Source: CAD feature listing. Evaluate the final solid. Frame: model axes, mm. Face numbers are marked on the shaded views. A direction names the side the tool comes from. Give positions to 0.01 mm unless a question says otherwise; leave off trailing zeros. Write each loop counter-clockwise with the first axis right and the second up, starting at its lowest first coordinate (ties: lowest second). Pieces come first, ordered by that corner, then holes. Notation, with made-up numbers: M 40.25,69 L 69.25,69 A31 ccw 69.25,105 Z; hole C 72.5,4 d4. An arc over 180 degrees is marked long. Return JSON: item names as keys, results as strings.
```python
from build123d import *

# Parameters (mm, degrees)
EXTRUDE_1_DEPTH     = 12
SKETCH_2_R          = 8
EXTRUDE_2_DEPTH     = 22
SKETCH_3_R          = 4.5
CUT_EXTRUDE_3_DEPTH = 39.626415832
CHAMFER_1_SIZE      = 1
CHAMFER_2_SIZE      = 1


with BuildPart() as part:
    # 草图1 → 拉伸1 (new body)
    with BuildSketch(Plane.XY):
        Polygon((-6.92820323, -12), (6.92820323, -12), (13.856406461, 0), (6.92820323, 12), (-6.92820323, 12), (-13.856406461, 0), align=None)
    extrude(amount=EXTRUDE_1_DEPTH)

    # 草图2 → 拉伸2 (add)
    with BuildSketch(Plane.XY.offset(12)):
        Circle(SKETCH_2_R)
    extrude(amount=EXTRUDE_2_DEPTH)

    # 草图3 → 拉伸3 (cut, through all)
    with BuildSketch(Plane(origin=(0, 0, 0), x_dir=(-1, 0, 0), z_dir=(0, 0, -1))):
        Circle(SKETCH_3_R)
    extrude(amount=-CUT_EXTRUDE_3_DEPTH, mode=Mode.SUBTRACT)

    # 倒角1
    chamfer_1_edges = [part.edges().sort_by_distance(p)[0] for p in [
        (-8, 0, 34),
    ]]
    chamfer(chamfer_1_edges, length=CHAMFER_1_SIZE)

    # 倒角2
    chamfer_2_edges = [part.edges().sort_by_distance(p)[0] for p in [
        (4.5, 0, 34),
    ]]
    chamfer(chamfer_2_edges, length=CHAMFER_2_SIZE)


solid = part.part
```
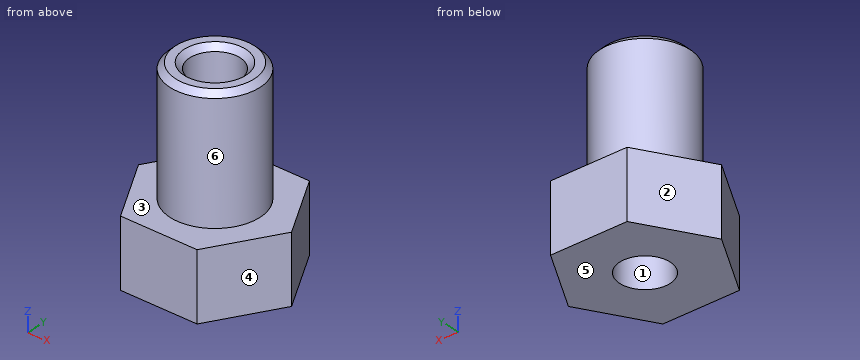
1) Draft query along Y for the marked faces 1, 2, 3 and 4. Return one class per face: released by +Y, released by -Y, zero draft, split by the parting line, or undercut.
Numbers:
{"face 1": "undercut", "face 2": "released by +Y", "face 3": "zero draft", "face 4": "released by -Y"}
2) Contact query for flat-ended pins moving along their axis: pin 1 Ø8 at (x, z) = (-4.5, 19.5) entering from +Y; pin 2 Ø8 at (x, z) = (-5.5, 22.5) entering from -Y; pin 3 Ø1.5 at (y, z) = (-8, 12.5) entering from -X. Output: stop coordinate, or through.
Numbers:
{"pin 1": "stops at y = 7.98", "pin 2": "stops at y = -7.86", "pin 3": "stops at x = -9.56"}
3) Cut plane B-B, the plane z = 7.5. Return the cut outline in (x, y), then the cut area to 3 significant figures.
Numbers:
{"outline": "M -13.86,0 L -6.93,-12 L 6.93,-12 L 13.86,0 L 6.93,12 L -6.93,12 Z; hole C 0,0 d9", "area": "435 mm²"}
4) Line query: line 1 (Y direction, x = 0, z = 17); line 2 (Z direction, x = -8.75, y = 4); line 3 (Y direction, x = 3.5, z = 4). Output: solid intervals per line, ascending. Write a range as [from, to].
Numbers:
{"line 1": "y = [-8, -4.5], [4.5, 8]", "line 2": "z = [0, 12]", "line 3": "y = [-12, -2.83], [2.83, 12]"}
5) Set-up query: the marked faces 5 and 6. Return all of +Z, -Z, +X, -X, +Y, -Y with unobstructed straight access to the full face (end or side cutting, diameter ignored); none if empty.
Numbers:
{"face 5": "-Z, +X, -X, +Y, -Y", "face 6": "+Z"}
6) Cut plane C-C, the plane x = -12. Return the cut outline in (y, z), then the cut area to 3 significant figures.
Numbers:
{"outline": "M -3.22,0 L 3.22,0 L 3.22,12 L -3.22,12 Z", "area": "77.2 mm²"}
7) Cut plane A-A, the plane x = 0. Return the cut outline in (y, z), then the cut area to 3 significant figures.
Numbers:
{"outline": "M -12,0 L -4.5,0 L -4.5,33 L -5.5,34 L -7,34 L -8,33 L -8,12 L -12,12 Z; M 4.5,0 L 12,0 L 12,12 L 8,12 L 8,33 L 7,34 L 5.5,34 L 4.5,33 Z", "area": "332 mm²"}
